```python
from build123d import *

# Parameters (mm, degrees)
SKETCH1_R                        = 12
BOSS_EXTRUDE1_DEPTH              = 100
SKETCH2_W                        = 140
SKETCH2_H                        = 90
CUT_EXTRUDE1_DEPTH               = 790.382670192
CUT_EXTRUDE2_START               = 225
SKETCH3_W                        = 47.5
SKETCH3_H                        = 80
SKETCH3_W_2                      = 102.5
SKETCH3_W_3                      = 150
CUT_EXTRUDE2_DEPTH               = 150
FILLET2_R                        = 10
FILLET4_R                        = 10
CHAMFER1_SIZE                    = 10
M24X2_0_TAPPED_HOLE1_D           = 22
M24X2_0_TAPPED_HOLE1_CSINK_D     = 24.05
M24X2_0_TAPPED_HOLE1_CSINK_ANGLE = 90
BOSS_EXTRUDE3_START              = -36
SKETCH7_R                        = 12
BOSS_EXTRUDE3_DEPTH              = 28


with BuildPart() as part:
    # Sketch1 → Boss-Extrude1 (new body)
    with BuildSketch(Plane(origin=(0, 0, 0), x_dir=(1, 0, 0), z_dir=(0, 1, 0))):
        Polygon((-375, 75), (375, 75), (375, -75), (-225, -75), (-225, -225), (-375, -225), (-375, -75), align=None)
        with Locations(Location((-300, -150, 0), (0, 0, 270))):
            Circle(SKETCH1_R, mode=Mode.SUBTRACT)
    extrude(amount=BOSS_EXTRUDE1_DEPTH)

    # Sketch2 → Cut-Extrude1 (cut, through all)
    with BuildSketch(Plane(origin=(375, 0, 0), x_dir=(0, 0, -1), z_dir=(1, 0, 0))):
        with Locations((0, 50)):
            Rectangle(SKETCH2_W, SKETCH2_H)
    extrude(amount=-CUT_EXTRUDE1_DEPTH, mode=Mode.SUBTRACT)

    # Sketch3 → Cut-Extrude2 (cut)
    with BuildSketch(Plane.ZY.offset(CUT_EXTRUDE2_START)):
        with Locations((351.25, 50)):
            Rectangle(SKETCH3_W, SKETCH3_H)
        with Locations((276.25, 50)):
            Rectangle(SKETCH3_W_2, SKETCH3_H)
        with Locations((150, 50)):
            Rectangle(SKETCH3_W_3, SKETCH3_H)
    extrude(amount=CUT_EXTRUDE2_DEPTH, mode=Mode.SUBTRACT)

    # Fillet2
    fillet2_edges = [part.edges().sort_by_distance(p)[0] for p in [
        (0, 100, -75),
        (0, 0, -75),
    ]]
    fillet(fillet2_edges, radius=FILLET2_R)

    # Fillet4
    fillet4_edges = [part.edges().sort_by_distance(p)[0] for p in [
        (75, 100, 75),
        (75, 0, 75),
    ]]
    fillet(fillet4_edges, radius=FILLET4_R)

    # Chamfer1
    chamfer1_edges = [part.edges().sort_by_distance(p)[0] for p in [
        (-225, 95, 225),
        (-375, 95, 225),
        (-225, 5, 225),
        (-375, 5, 225),
    ]]
    chamfer(chamfer1_edges, length=CHAMFER1_SIZE)

    # M24x2.0 Tapped Hole1 (through all)
    with Locations(Plane(origin=(0, 100, 0), x_dir=(1, 0, 0), z_dir=(0, 1, 0))):
        with Locations((100, 0), (325, 0), (-125, 0)):
            CounterSinkHole(M24X2_0_TAPPED_HOLE1_D / 2, M24X2_0_TAPPED_HOLE1_CSINK_D / 2, counter_sink_angle=M24X2_0_TAPPED_HOLE1_CSINK_ANGLE)

    # Sketch7 → Boss-Extrude3 (add)
    with BuildSketch(Plane(origin=(0, 100, 0), x_dir=(1, 0, 0), z_dir=(0, 1, 0)).offset(BOSS_EXTRUDE3_START)):
        with BuildLine():
            Line((-81.456914067, -75), (-51.717949801, -115))
            ThreePointArc((-51.717949801, -115), (-31.456914067, -125.183627997), (-11.195878332, -115))
            Line((-11.195878332, -115), (18.543085933, -75))
            Line((18.543085933, -75), (-81.456914067, -75))
        make_face()
        with Locations(Location((-31.456914067, -97.533391436, 0), (0, 0, 270))):
            Circle(SKETCH7_R, mode=Mode.SUBTRACT)
    extrude(amount=-BOSS_EXTRUDE3_DEPTH)


solid = part.part
```
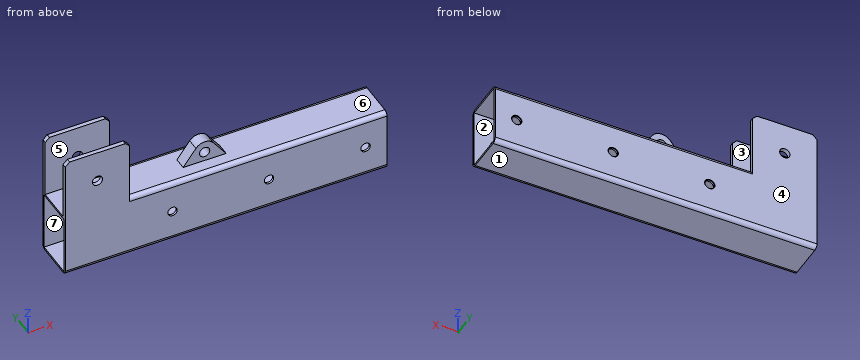
Work out the finished part from the listing and answer in its coordinate system (mm). Face numbers are marked on the shaded views. A direction names the side the tool comes from. Give positions to 0.01 mm unless a question says otherwise; leave off trailing zeros. Write each loop counter-clockwise with the first axis right and the second up, starting at its lowest first coordinate (ties: lowest second). Pieces come first, ordered by that corner, then holes.
(1) The mould has two halves that part along Z. Classify the marked faces 1, 2 and 3: pulls with the +Z half, pulls with the -Z half, needs draft (parallel to the pull), parting line crosses it, or undercut.
Final values:
face 1: pulls with the -Z half
face 2: undercut
face 3: needs draft
(2) The part is cut by section D-D on z = 36. Write down the section's boundary in (x, y).
Final values:
outline: (-375, 0) - (375, 0) - (375, 5) - (-375, 5) - close; (-375, 95) - (375, 95) - (375, 100) - (-375, 100) - close
(3) Which of the six approach directions +Z, -Z, +X, -X, +Y, -Y give full straight-line access (tool end or side, diameter ignored) to the marked faces 4, 5, 6 and 7?
Final values:
face 4: +Z, -Z, +X, -X, +Y
face 5: +Z, +X, -X
face 6: +Z
face 7: +X, -X
(4) Straight lines are drawn through the part: line 1 (Y direction, x = 217, z = 35); line 2 (Z direction, x = 169.5, y = 85); line 3 (Y direction, x = -243, z = 160). For each, find the intervals that lie inside material, in ascending order.
Final values:
line 1: y = 0 to 5, 95 to 100
line 2: z = -75 to -70, 70 to 75
line 3: y = 0 to 10, 90 to 100
(5) The part is cut by section B-B on z = 150. Write down the section's boundary in (x, y), plus the area to 3 significant figures.
Final values:
outline: (-375, 0) - (-312, 0) - (-312, 10) - (-375, 10) - close; (-375, 90) - (-312, 90) - (-312, 100) - (-375, 100) - close; (-288, 0) - (-225, 0) - (-225, 10) - (-288, 10) - close; (-288, 90) - (-225, 90) - (-225, 100) - (-288, 100) - close
area: 2,520 mm2
(6) The part is cut by section A-A on x = -300. Write down the section's boundary in (y, z), plus the area to 3 significant figures.
Final values:
outline: (0, -65) arc R10 ccw to (10, -75) - (90, -75) arc R10 ccw to (100, -65) - (100, 138) - (90, 138) - (90, 75) - (10, 75) - (10, 138) - (0, 138) - close; (0, 162) - (10, 162) - (10, 225) - (0, 225) - close; (90, 162) - (100, 162) - (100, 225) - (90, 225) - close; hole (5, -70) - (95, -70) - (95, 70) - (5, 70) - close
area: 4,880 mm2
(7) Flat-ended cylindrical pins translate along their axes: pin 1 Ø4 at (x, z) = (200.5, 74) entering from +Y; pin 2 Ø4 at (x, y) = (43.5, 30.5) entering from +Z; pin 3 Ø19 at (x, z) = (-300, 150) entering from +Y; pin 4 Ø25 at (x, z) = (-34.5, 98.5) entering from +Y. Find the tip coordinate at first contact, or state that the pin passes through.
Final values:
pin 1: stops at y = 97.14
pin 2: stops at z = 75
pin 3: passes through
pin 4: stops at y = 64
(8) The part is cut by section C-C on x = 143.5. Write down the section's boundary in (y, z).
Final values:
outline: (0, -65) arc R10 ccw to (10, -75) - (90, -75) arc R10 ccw to (100, -65) - (100, 65) arc R10 ccw to (90, 75) - (10, 75) arc R10 ccw to (0, 65) - close; hole (5, -70) - (95, -70) - (95, 70) - (5, 70) - close
